Read the model definition and answer for the solid it produces. Units are mm, in the model's axes. Give positions to 0.01 mm unless a question says otherwise; leave off trailing zeros. Loops run counter-clockwise (first coordinate to the right, second up) from the corner with the lowest first, then second, coordinate; pieces in that order, holes last. Notation, with made-up numbers: (16, 38) - (31, 38) arc R21 cw to (31, 52) - close; hole circle Ø9 at (33, 77.25). An arc over 180 degrees is marked (long way). Write item = value, one per line.
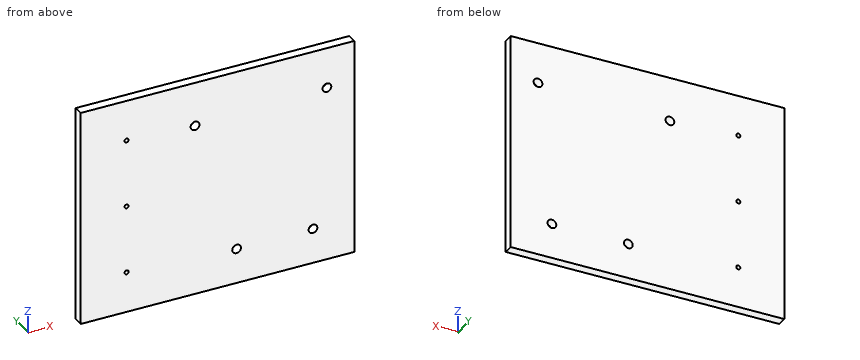
```python
from build123d import *

# Parameters (mm, degrees)
SKETCH1_W           = 100
SKETCH1_H           = 80
BOSS_EXTRUDE1_DEPTH = 3.5
SKETCH2_R           = 1.6
SKETCH2_R_2         = 0.75
CUT_EXTRUDE1_DEPTH  = 65.126827459


with BuildPart() as part:
    # Sketch1 → Boss-Extrude1 (new body)
    with BuildSketch(Plane(origin=(0, 0, 0), x_dir=(1, 0, 0), z_dir=(0, 1, 0))):
        Rectangle(SKETCH1_W, SKETCH1_H)
    extrude(amount=BOSS_EXTRUDE1_DEPTH)

    # Sketch2 → Cut-Extrude1 (cut, through all)
    with BuildSketch(Plane(origin=(0, 3.5, 0), x_dir=(1, 0, 0), z_dir=(0, 1, 0))):
        with Locations(Location((40, -25, 0), (0, 0, 270))):
            Circle(SKETCH2_R)
        with Locations(Location((-8.2, -23.7, 0), (0, 0, 270))):
            Circle(SKETCH2_R)
        with Locations(Location((7, 27.1, 0), (0, 0, 270))):
            Circle(SKETCH2_R)
        with Locations(Location((34.9, 27.1, 0), (0, 0, 270))):
            Circle(SKETCH2_R)
        with Locations(Location((-33.2, -25, 0), (0, 0, 270))):
            Circle(SKETCH2_R_2)
        with Locations(Location((-33.2, 25, 0), (0, 0, 90))):
            Circle(SKETCH2_R_2)
        with Locations(Location((-33.2, 0, 0), (0, 0, 270))):
            Circle(SKETCH2_R_2)
    extrude(amount=-CUT_EXTRUDE1_DEPTH, mode=Mode.SUBTRACT)


solid = part.part
```
1) Find the intervals of material crossed by probe 1 along Z at (x, y) = (-33.2, 1.3); probe 2 along X at (y, z) = (1.2, -27.1); probe 3 along X at (y, z) = (2.65, 25), in increasing order.
Output:
probe_1 = -40 to -25.75, -24.25 to -0.75, 0.75 to 24.25, 25.75 to 40
probe_2 = -50 to 5.4, 8.6 to 33.3, 36.5 to 50
probe_3 = -50 to -33.95, -32.45 to -9.13, -7.27 to 38.4, 41.6 to 50
2) A cutting plane is placed at B-B on x = 34.9. Determine the outline of the cut face in (y, z), then the cut area to 3 significant figures.
Output:
outline = (0, -40) - (3.5, -40) - (3.5, -28.7) - (0, -28.7) - close; (0, -25.5) - (3.5, -25.5) - (3.5, 40) - (0, 40) - close
area = 269 mm²
3) A cutting plane is placed at A-A on z = -27.1. Determine the outline of the cut face in (x, y).
Output:
outline = (-50, 0) - (5.4, 0) - (5.4, 3.5) - (-50, 3.5) - close; (8.6, 0) - (33.3, 0) - (33.3, 3.5) - (8.6, 3.5) - close; (36.5, 0) - (50, 0) - (50, 3.5) - (36.5, 3.5) - close
